from build123d import *

# Parameters (mm, degrees)
SKETCH_1_R          = 11.25
EXTRUDE_1_DEPTH     = 35.5
SKETCH_2_R          = 3.75
EXTRUDE_2_DEPTH     = 14.5
FILLET_1_R          = 3
SKETCH_3_R          = 1.5
CUT_EXTRUDE_1_DEPTH = 10


with BuildPart() as part:
    # 草圖1 → 填料-伸長1 (new body)
    with BuildSketch(Plane.XY):
        Circle(SKETCH_1_R)
    extrude(amount=EXTRUDE_1_DEPTH)

    # 草圖2 → 填料-伸長2 (add)
    with BuildSketch(Plane.XY.offset(35.5)):
        Circle(SKETCH_2_R)
    extrude(amount=EXTRUDE_2_DEPTH)

    # 圓角1
    fillet_1_edges = [part.edges().sort_by_distance(p)[0] for p in [
        (-3.75, 0, 35.5),
    ]]
    fillet(fillet_1_edges, radius=FILLET_1_R)

    # 草圖3 → 除料-伸長1 (cut)
    with BuildSketch(Plane(origin=(0, 0, 0), x_dir=(-1, 0, 0), z_dir=(0, 0, -1))):
        with Locations((-8.5, 0)):
            Circle(SKETCH_3_R)
        with Locations((8.5, 0)):
            Circle(SKETCH_3_R)
        with Locations((0, -8.5)):
            Circle(SKETCH_3_R)
        with Locations((0, 8.5)):
            Circle(SKETCH_3_R)
    extrude(amount=-CUT_EXTRUDE_1_DEPTH, mode=Mode.SUBTRACT)


solid = part.part
The listing builds one solid part. Answer for the finished solid, in the listing's coordinates (mm). A direction names the side the tool comes from. Round coordinates to 2 decimals unless told otherwise and drop trailing zeros. Loops run counter-clockwise (first coordinate to the right, second up) from the corner with the lowest first, then second, coordinate; pieces in that order, holes last. Notation, with made-up numbers: M -23,24.5 L 10,24.5 A13 ccw 10,34.5 Z; hole C 83,33 d6. An arc over 180 degrees is marked long. Return JSON: item names as keys, results as strings.
Q1. Each of these flat-tipped pins is pushed along its axis until it touches: pin 1 Ø0.9 at (x, y) = (8, -0.5) entering from -Z; pin 2 Ø2.5 at (x, y) = (0, 8.5) entering from +Z; pin 3 Ø3 at (x, z) = (-6.5, 9.5) entering from -Y; pin 4 Ø6 at (x, y) = (4.5, 6) entering from -Z. Where does it stop, or does it pass through?
Results list:
{"pin 1": "stops at z = 10", "pin 2": "stops at z = 35.5", "pin 3": "stops at y = -10.08", "pin 4": "stops at z = 0"}
Q2. Find section A-A, the plane z = 9. Determine the outline of the cut face in (x, y).
Results list:
{"outline": "C 0,0 d22.5; hole C -8.5,0 d3; hole C 0,-8.5 d3; hole C 0,8.5 d3; hole C 8.5,0 d3"}
Q3. Find section B-B, the plane x = 0. Determine the outline of the cut face in (y, z).
Results list:
{"outline": "M -11.25,0 L -10,0 L -10,10 L -7,10 L -7,0 L 7,0 L 7,10 L 10,10 L 10,0 L 11.25,0 L 11.25,35.5 L 6.75,35.5 A3 cw 3.75,38.5 L 3.75,50 L -3.75,50 L -3.75,38.5 A3 cw -6.75,35.5 L -11.25,35.5 Z"}
Q4. Find the intervals of material crossed by line 1 along Y through (x, z) = (0, 5); line 2 along Z through (x, y) = (7.5, 1.75); line 3 along Y through (x, z) = (8.5, 4), in increasing order. Write a range as from..to.
Results list:
{"line 1": "y = -11.25..-10, -7..7, 10..11.25", "line 2": "z = 0..35.5", "line 3": "y = -7.37..-1.5, 1.5..7.37"}
Q5. The mould has two halves that part along Y. Classify faces 3 (the face through (10, 0, 5)), 4 (the face through (-3.746, 0.165, 44.17)), 5 (the face through (5, -5, 35.5)): released by +Y, released by -Y, zero draft, split by the parting line, or undercut.
Results list:
{"face 3": "undercut", "face 4": "split by the parting line", "face 5": "zero draft"}
Q6. Find section C-C, the plane y = 7.75. Determine the outline of the cut face in (x, z), plus the area to 3 significant figures.
Results list:
{"outline": "M -8.15,0 L -1.3,0 L -1.3,10 L 1.3,10 L 1.3,0 L 8.15,0 L 8.15,35.5 L -8.15,35.5 Z", "area": "553 mm2"}
Q7. Which of the six approach directions +Z, -Z, +X, -X, +Y, -Y give full straight-line access (tool end or side, diameter ignored) to faces 1 (the face through (-8, 0, 10)), 2 (the face through (0, 0, 50))?
Results list:
{"face 1": "-Z", "face 2": "+Z, +X, -X, +Y, -Y"}
Q8. Find section D-D, the plane z = 40.5. Determine the outline of the cut face in (x, y), plus the area to 3 significant figures.
Results list:
{"outline": "C 0,0 d7.5", "area": "44.2 mm2"}
